Part model, mm, in its own coordinate system. Face numbers are marked on the shaded views. A direction names the side the tool comes from. Give positions to 0.01 mm unless a question says otherwise; leave off trailing zeros. Loops run counter-clockwise (first coordinate to the right, second up) from the corner with the lowest first, then second, coordinate; pieces in that order, holes last. Notation, with made-up numbers: M 68.25,57.25 L 101.25,57.25 A34 ccw 101.25,95.25 Z; hole C 72.5,86.25 d5. An arc over 180 degrees is marked long. Answer in a Markdown table with one row per item.
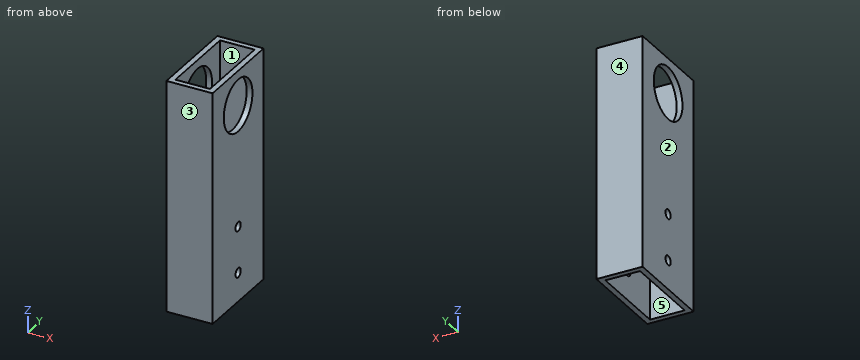
Autodesk Inventor part; units mm, degrees
ref_plane "YZ Plane" through (0, 0, 0) normal (1, 0, 0) x (0, 1, 0)
ref_plane "XZ Plane" through (0, 0, 0) normal (0, 1, 0) x (-1, 0, 0)
ref_plane "XY Plane" through (0, 0, 0) normal (0, 0, 1) x (1, 0, 0)
sketch "Sketch1" plane through (0, 0, 0) normal (0, 0, 1) x (1, 0, 0)
  line L0 (-6.6707, 4.0865) -> (18.7293, 4.0865)
  line L1 (18.7293, 4.0865) -> (18.7293, -46.7135)
  line L2 (18.7293, -46.7135) -> (-6.6707, -46.7135)
  line L3 (-6.6707, -46.7135) -> (-6.6707, 4.0865)
  line L4 (15.5543, 0.9115) -> (-3.4957, 0.9115)
  line L5 (-3.4957, 0.9115) -> (-3.4957, -43.5385)
  line L6 (-3.4957, -43.5385) -> (15.5543, -43.5385)
  line L7 (15.5543, -43.5385) -> (15.5543, 0.9115)
  point P0 (0, 0)
  dimension "d0" = 25.4
  dimension "d1" = 50.8
  dimension "d2" = 3.175
extrude "Extrusion1" add sketch "Sketch1" along normal blind 127
sketch "Sketch2" plane through (18.7293, -46.7135, 0) normal (1, 0, 0) x (0, 0, -1)
  line L0 (0, 47.625) -> (0, 3.175)
  line L1 (0, 25.4) -> (-107.95, 25.4)
  circle A0 centre (-107.95, 25.4) radius 14.2875
  point P0 (0, 46.7135)
  dimension "d5" = 107.95
  dimension "d6" = 28.575
extrude "Extrusion2" cut sketch "Sketch2" against normal blind 101.6
sketch "Sketch3" plane through (18.7293, -46.7135, 0) normal (1, 0, 0) x (0, 0, -1)
  line L0 (0, 47.625) -> (0, 3.175)
  line L1 (0, 25.4) -> (-15.875, 25.4)
  line L2 (-15.875, 25.4) -> (-41.275, 25.4)
  circle A0 centre (-15.875, 25.4) radius 2.5797
  circle A1 centre (-41.275, 25.4) radius 2.5797
  point P0 (0, 46.7135)
  dimension "d9" = 15.875
  dimension "d10" = 25.4
  dimension "d11" = 5.1594
  dimension "d12" = 5.1594
extrude "Extrusion3" cut sketch "Sketch3" against normal blind 101.6
properties part number "Gearbox Shaft Stabilizer"
(1) Drill centre lines: line 1 along Y through (x, z) = (12.25, 75.5); line 2 along Y through (x, z) = (-4.35, 107.95); line 3 along X through (y, z) = (-37, 21.5). Where is each one in solid material? Low to high.
Recorded:
| item | result |
|---|---|
| line 1 | y = -46.71 to -43.54, 0.91 to 4.09 |
| line 2 | y = -46.71 to -35.6, -7.03 to 4.09 |
| line 3 | x = -6.67 to -3.5, 15.55 to 18.73 |
(2) Which spindle directions (+Z, -Z, +X, -X, +Y, -Y) get a long thin tool onto all of the face, cutting with end or side? Do the marked faces 4 and 5. Say none if no direction does.
Recorded:
| item | result |
|---|---|
| face 4 | +Z, -Z, +X, -X, +Y |
| face 5 | +Z, -Z |
(3) Pin check, flat tip, straight feed: pin 1 Ø1.5 at (x, y) = (-2, -3) entering from +Z (1 decimal). Stop position of the tip, or through.
Recorded:
| item | result |
|---|---|
| pin 1 | passes through |
(4) Saw through at B-B (y = -1.5). Write the cut outline in (x, z), plus the area to 3 significant figures.
Recorded:
| item | result |
|---|---|
| outline | M -6.67,0 L -3.5,0 L -3.5,127 L -6.67,127 Z; M 15.55,0 L 18.73,0 L 18.73,127 L 15.55,127 Z |
| area | 806 mm^2 |
(5) Saw through at A-A (z = 107.95). Write the cut outline in (x, y).
Recorded:
| item | result |
|---|---|
| outline | M -6.67,-46.71 L 18.73,-46.71 L 18.73,-35.6 L 15.55,-35.6 L 15.55,-43.54 L -3.5,-43.54 L -3.5,-35.6 L -6.67,-35.6 Z; M -6.67,-7.03 L -3.5,-7.03 L -3.5,0.91 L 15.55,0.91 L 15.55,-7.03 L 18.73,-7.03 L 18.73,4.09 L -6.67,4.09 Z |
(6) Saw through at D-D (z = 9). Write the cut outline in (x, y), plus the area to 3 significant figures.
Recorded:
| item | result |
|---|---|
| outline | M -6.67,-46.71 L 18.73,-46.71 L 18.73,4.09 L -6.67,4.09 Z; hole M -3.5,-43.54 L 15.55,-43.54 L 15.55,0.91 L -3.5,0.91 Z |
| area | 444 mm^2 |
(7) Pull direction X, two halves, no side cores. Call the marked faces 1, 2 and 3: +X half, -X half, draft (parallel to the pull), parting line (faces both ways), or undercut.
Recorded:
| item | result |
|---|---|
| face 1 | undercut |
| face 2 | -X half |
| face 3 | draft |
(8) Saw through at C-C (x = 4.5). Write the cut outline in (y, z), plus the area to 3 significant figures.
Recorded:
| item | result |
|---|---|
| outline | M -46.71,0 L -43.54,0 L -43.54,127 L -46.71,127 Z; M 0.91,0 L 4.09,0 L 4.09,127 L 0.91,127 Z |
| area | 806 mm^2 |
